Verification items for the finished model (mm, model axes). Face numbers are marked on the shaded views. A direction names the side the tool comes from. Give positions to 0.01 mm unless a question says otherwise; leave off trailing zeros. Loops run counter-clockwise (first coordinate to the right, second up) from the corner with the lowest first, then second, coordinate; pieces in that order, holes last. Notation, with made-up numbers: (87, 75) - (121, 75) arc R16 ccw to (121, 99) - close; hole circle Ø1 at (71, 46). An arc over 180 degrees is marked (long way). Answer in a Markdown table with one row per item.
```python
from build123d import *

# Parameters (mm, degrees)
CROQUIS1_W              = 16.5
CROQUIS1_H              = 16.5
CROQUIS1_W_2            = 12.5
CROQUIS1_H_2            = 12.5
SALIENTE_EXTRUIR1_DEPTH = 10
CHAFL_N1_SIZE           = 2
CROQUIS2_W              = 16.5
CROQUIS2_H              = 2
SALIENTE_EXTRUIR2_DEPTH = 12.5
REDONDEO1_R             = 1


with BuildPart() as part:
    # Croquis1 → Saliente-Extruir1 (new body)
    with BuildSketch(Plane(origin=(0, 0, 0), x_dir=(1, 0, 0), z_dir=(0, 1, 0))):
        Rectangle(CROQUIS1_W, CROQUIS1_H)
        Rectangle(CROQUIS1_W_2, CROQUIS1_H_2, mode=Mode.SUBTRACT)
    extrude(amount=SALIENTE_EXTRUIR1_DEPTH)

    # Chaflán1
    chafl_n1_edges = [part.edges().sort_by_distance(p)[0] for p in [
        (6.25, 10, 0),
    ]]
    chamfer(chafl_n1_edges, length=CHAFL_N1_SIZE - 0.0001)  # a hair under: the kernel refuses the full size

    # Croquis2 → Saliente-Extruir2 (add)
    with BuildSketch(Plane(origin=(8.25, 0, 0), x_dir=(0, 0, -1), z_dir=(1, 0, 0))):
        with Locations((0, 9)):
            Rectangle(CROQUIS2_W, CROQUIS2_H)
    extrude(amount=SALIENTE_EXTRUIR2_DEPTH)

    # Redondeo1
    redondeo1_edges = [part.edges().sort_by_distance(p)[0] for p in [
        (-6.25, 5, -6.25),
        (-6.25, 5, 6.25),
        (8.25, 4, -8.25),
        (8.25, 4, 8.25),
        (20.75, 9, 8.25),
        (20.75, 9, -8.25),
        (-8.25, 5, -8.25),
        (-8.25, 5, 8.25),
    ]]
    fillet(redondeo1_edges, radius=REDONDEO1_R)


solid = part.part
```
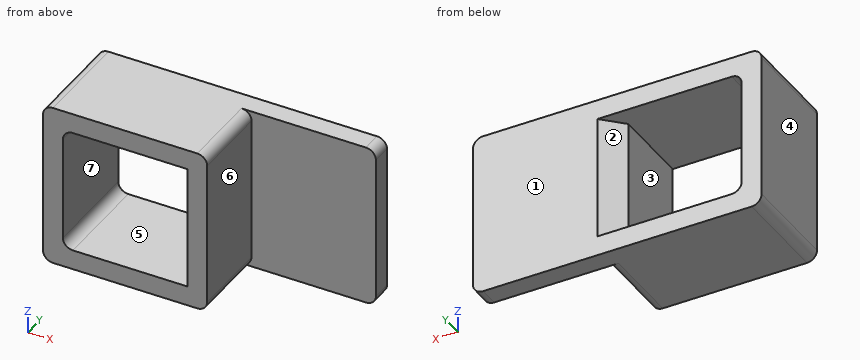
Q1. Sectioned sample at C-C (z = -4.75). Record the cut outline in (x, y).
Completed:
| item | result |
|---|---|
| outline | (-8.25, 0) - (-6.25, 0) - (-6.25, 10) - (-8.25, 10) - close; (6.25, 0) - (8.25, 0) - (8.25, 8) - (20.75, 8) - (20.75, 10) - (8.25, 10) - (6.25, 8) - close |
Q2. Draft check along X on the marked faces 4, 5, 6 and 7. Enter one of: +X half, -X half, draft (parallel to the pull), parting line (faces both ways), or undercut.
Completed:
| item | result |
|---|---|
| face 4 | -X half |
| face 5 | undercut |
| face 6 | +X half |
| face 7 | undercut |
Q3. Sectioned sample at A-A (x = -3.25). Record the cut outline in (y, z).
Completed:
| item | result |
|---|---|
| outline | (0, -8.25) - (10, -8.25) - (10, -6.25) - (0, -6.25) - close; (0, 6.25) - (10, 6.25) - (10, 8.25) - (0, 8.25) - close |
Q4. Go/stop test with flat-tipped pins: P1, Ø3, axis at y = 3.5, z = -2, coming from the +X side; P2, Ø1, axis at x = 11, z = 3, coming from the -Y side. Record where each tip stops, or that it passes through.
Completed:
| item | result |
|---|---|
| P1 | x = 8.25 |
| P2 | y = 8 |
Q5. Thickness scan on line 1 (X direction, y = 3, z = -1.25); line 2 (Y direction, x = 10.5, z = 1.5). Record the ranges inside material, lowest first.
Completed:
| item | result |
|---|---|
| line 1 | -8.25 to -6.25, 6.25 to 8.25 |
| line 2 | 8 to 10 |
Q6. Tool access check on the marked faces 1, 2 and 3. Record the directions out of +Z, -Z, +X, -X, +Y, -Y that give a thin tool (end or side, any length) a straight path to the whole face; none if there is none.
Completed:
| item | result |
|---|---|
| face 1 | +Z, -Z, +X, -X, +Y |
| face 2 | +Y |
| face 3 | +Y, -Y |
Q7. Sectioned sample at B-B (y = 1.5). Record the cut outline in (x, z), and give its area (3 significant figures).
Completed:
| item | result |
|---|---|
| outline | (-8.25, -7.25) arc R1 ccw to (-7.25, -8.25) - (7.25, -8.25) arc R1 ccw to (8.25, -7.25) - (8.25, 7.25) arc R1 ccw to (7.25, 8.25) - (-7.25, 8.25) arc R1 ccw to (-8.25, 7.25) - close; hole (-6.25, -5.25) arc R1 ccw to (-5.25, -6.25) - (6.25, -6.25) - (6.25, 6.25) - (-5.25, 6.25) arc R1 ccw to (-6.25, 5.25) - close |
| area | 116 mm^2 |
Q8. Sectioned sample at D-D (x = 18). Record the cut outline in (y, z), and give its area (3 significant figures).
Completed:
| item | result |
|---|---|
| outline | (8, -8.25) - (10, -8.25) - (10, 8.25) - (8, 8.25) - close |
| area | 33.0 mm^2 |
